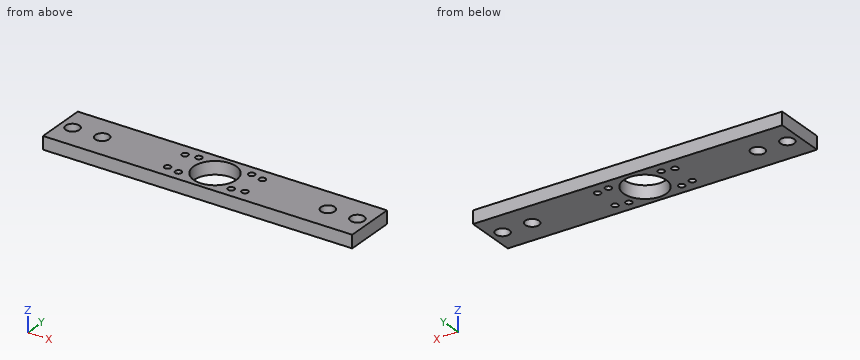
Autodesk Inventor part; units mm, degrees
ref_plane "Work Plane1" through (-30.9265, 0, 3.175) normal (0, -1, 0) x (1, 0, 0)
ref_plane "Work Plane2" through (0, 12.6269, 3.175) normal (-1, 0, 0) x (0, -1, 0)
ref_plane "YZ Plane" through (0, 0, 0) normal (1, 0, 0) x (0, 1, 0)
sketch "Sketch1" plane through (0, 0, 0) normal (0, 0, 1) x (1, 0, 0)
  circle A0 centre (0, 0) radius 6.477 construction
  circle A1 centre (0, 0) radius 4.75 construction
  circle A2 centre (0, 0) radius 9.525 construction
  line L0 (-38.1, -6.35) -> (38.1, -6.35) construction
  line L1 (38.1, -6.35) -> (38.1, 6.35) construction
  line L2 (38.1, 6.35) -> (-38.1, 6.35) construction
  line L3 (-38.1, 6.35) -> (-38.1, -6.35) construction
  line L4 (-38.1, 6.35) -> (38.1, 6.35)
  line L5 (38.1, 6.35) -> (38.1, -6.35)
  line L6 (38.1, -6.35) -> (-38.1, -6.35)
  line L7 (-38.1, -6.35) -> (-38.1, 6.35)
  dimension "d0" = 12.954
  dimension "d1" = 9.5
  dimension "d2" = 19.05
  dimension "d3" = 76.2
  dimension "d4" = 12.7
extrude "Extrusion1" add sketch "Sketch1" along normal blind 3.175
sketch "Sketch2" plane through (0, 0, 3.175) normal (0, 0, 1) x (1, 0, 0)
  circle A0 centre (0, 0) radius 5.25
  dimension "d7" = 10.5
extrude "Extrusion2" cut sketch "Sketch2" against normal through all
sketch "Sketch4" plane through (0, 0, 3.175) normal (0, 0, 1) x (1, 0, 0)
  circle A0 centre (0, 0) radius 5.25
  circle A1 centre (0, 0) radius 7.5 construction
  arc A2 (6.4952, 3.75) -> (-6.4952, 3.75) centre (0, 0) ccw construction
  line L0 (0, 0) -> (6.4952, 3.75) construction
  line L1 (0, 0) -> (7.5, 0) construction
  line L2 (0, 0) -> (-6.4952, 3.75) construction
  point P0 (6.4952, 3.75)
  dimension "d13" = 15
  dimension "d14" = 30
  dimension "d15" = 120
hole "Hole1" at (-6.4952, 3.75, 3.175) at (6.4952, 3.75, 3.175) direction (0, 0, -1) diameter 1.5748 end through all
sketch "Sketch5" plane through (0, 0, 3.175) normal (0, 0, 1) x (1, 0, 0)
  circle A0 centre (6.4952, 3.75) radius 0.7874
  circle A1 centre (-6.4952, 3.75) radius 0.7874
  circle A2 centre (0, 0) radius 5.25
  line L0 (38.1, -6.35) -> (-38.1, -6.35)
  line L1 (38.1, 6.35) -> (38.1, -6.35)
  line L2 (-38.1, 6.35) -> (38.1, 6.35)
  line L3 (-38.1, -6.35) -> (-38.1, 6.35)
  line L4 (-30.9265, 0) -> (29.6642, 0) construction
ref_plane "Work Plane1" through (-30.9265, 0, 3.175) normal (0, -1, 0) x (1, 0, 0)
mirror "Mirror1" about plane through (-30.9265, 0, 3.175) normal (0, -1, 0) of "Hole1"
sketch "Sketch6" plane through (0, 0, 3.175) normal (0, 0, 1) x (1, 0, 0)
  line L0 (-35.1, 0) -> (-27.8102, 0)
  line L1 (-27.8102, 0) -> (-27.8102, 2.0321)
  line L2 (-27.8102, 2.0321) -> (-35.1, 2.0321)
  line L3 (-35.1, 2.0321) -> (-35.1, 0)
  line L4 (-38.1, -6.35) -> (-38.1, 6.35)
  dimension "d39" = 7.2898
  dimension "d40" = 3
hole "Hole2" at (-35.1, 0, 3.175) at (-27.8102, 0, 3.175) direction (0, 0, -1) diameter 3.4036 end through all
sketch "Sketch7" plane through (0, 0, 3.175) normal (0, 0, 1) x (1, 0, 0)
  circle A0 centre (-27.8102, 0) radius 1.7018
  circle A1 centre (-35.1, 0) radius 1.7018
  circle A2 centre (6.4952, -3.75) radius 0.7874
  circle A3 centre (-6.4952, -3.75) radius 0.7874
  circle A4 centre (6.4952, 3.75) radius 0.7874
  circle A5 centre (-6.4952, 3.75) radius 0.7874
  circle A6 centre (0, 0) radius 5.25
  line L0 (38.1, -6.35) -> (-38.1, -6.35)
  line L1 (38.1, 6.35) -> (38.1, -6.35)
  line L2 (-38.1, 6.35) -> (38.1, 6.35)
  line L3 (-38.1, -6.35) -> (-38.1, 6.35)
  line L4 (0, 12.6269) -> (0, -12.6269) construction
ref_plane "Work Plane2" through (0, 12.6269, 3.175) normal (-1, 0, 0) x (0, -1, 0)
mirror "Mirror2" about plane through (0, 12.6269, 3.175) normal (-1, 0, 0) of "Hole2"
sketch "Sketch8" plane through (0, 0, 3.175) normal (0, 0, 1) x (1, 0, 0)
  point P0 (-9.525, -3.175)
  point P1 (-9.525, 3.175)
  point P2 (9.525, 3.175)
  point P3 (9.525, -3.175)
hole "Hole3" at (-9.525, 3.175, 3.175) at (-9.525, -3.175, 3.175) at (9.525, -3.175, 3.175) at (9.525, 3.175, 3.175) direction (0, 0, -1) diameter 1.5748 end through all
properties part number "simple_chuck_force_bridge"
Here's how the part is built. I have some questions about the finished solid (model axes, mm). Give positions to 0.01 mm unless a question says otherwise; leave off trailing zeros. Write each loop counter-clockwise with the first axis right and the second up, starting at its lowest first coordinate (ties: lowest second). Pieces come first, ordered by that corner, then holes.
(1) Imagine slicing it at B-B, the plane x = 35.1. Write out the boundary of the cut face in (y, z) (3 decimals).
Output values:
outline: (-6.35, 0) - (-1.702, 0) - (-1.702, 3.175) - (-6.35, 3.175) - close; (1.702, 0) - (6.35, 0) - (6.35, 3.175) - (1.702, 3.175) - close
(2) If I drill on L1, parallel to Y at x = -9, z = 0.6; L2, parallel to X at y = -3.75, z = 1.25; L3, parallel to X at y = 2.75, z = 0.6, over which ranges is the centre line in solid material (lowest first)?
Output values:
L1: y = -6.35 to -3.76, -2.59 to 2.59, 3.76 to 6.35
L2: x = -38.1 to -10.06, -8.99 to -7.28, -5.71 to -3.67, 3.67 to 5.71, 7.28 to 8.99, 10.06 to 38.1
L3: x = -38.1 to -10.19, -8.86 to -4.47, 4.47 to 8.86, 10.19 to 38.1
(3) Imagine slicing it at C-C, the plane z = 1.65. Count the separate pieces of the cut face and the enclosed holes in it, and give its area (3 significant figures).
Output values:
separate pieces: 1
enclosed holes: 13
area: 829 mm2
(4) Imagine slicing it at D-D, the plane x = 0. Write out the boundary of the cut face in (y, z) (3 decimals).
Output values:
outline: (-6.35, 0) - (-5.25, 0) - (-5.25, 3.175) - (-6.35, 3.175) - close; (5.25, 0) - (6.35, 0) - (6.35, 3.175) - (5.25, 3.175) - close
(5) Imagine slicing it at A-A, the plane y = 0. Write out the boundary of the cut face in (x, z) (3 decimals), and give its area (3 significant figures).
Output values:
outline: (-38.1, 0) - (-36.802, 0) - (-36.802, 3.175) - (-38.1, 3.175) - close; (-33.398, 0) - (-29.512, 0) - (-29.512, 3.175) - (-33.398, 3.175) - close; (-26.108, 0) - (-5.25, 0) - (-5.25, 3.175) - (-26.108, 3.175) - close; (5.25, 0) - (26.108, 0) - (26.108, 3.175) - (5.25, 3.175) - close; (29.512, 0) - (33.398, 0) - (33.398, 3.175) - (29.512, 3.175) - close; (36.802, 0) - (38.1, 0) - (38.1, 3.175) - (36.802, 3.175) - close
area: 165 mm2
